from build123d import *

# Parameters (mm, degrees)
SKETCH1_W               = 6.35
SKETCH1_H               = 36.5125
CHAMFER2_SIZE           = 1.5875
SKETCH5_W               = 11.1125
SKETCH5_H               = 46.0375
CUT_EXTRUDE1_DEPTH      = 18.4625
CUT_EXTRUDE1_DEPTH_BACK = 18.4625
SKETCH6_R               = 12.3825
CUT_EXTRUDE2_DEPTH      = 7.3500001
CUT_EXTRUDE2_DEPTH_BACK = 7.3500001
SCALE1_SCALE            = 0.75
SCALE2_SCALE            = 0.666666667


with BuildPart() as part:
    # Sketch1 → Revolve1 (revolve)
    with BuildSketch(Plane.XY):
        with Locations((3.175, -18.25625)):
            Rectangle(SKETCH1_W, SKETCH1_H)
    revolve(axis=Axis((0, 46.0375, 0), (0, -1, 0)))

    # Chamfer2
    chamfer2_edges = [part.edges().sort_by_distance(p)[0] for p in [
        (-6.35, -36.5125, 0),
    ]]
    chamfer(chamfer2_edges, length=CHAMFER2_SIZE)

    # Sketch4 → Revolve2 (revolve)
    with BuildSketch(Plane.XY):
        with BuildLine():
            Line((6.35, 0), (0, 0))
            Line((0, 0), (0, 46.0375))
            ThreePointArc((0, 46.0375), (15.983688754, 35.607823052), (12.874497319, 16.77727882))
            ThreePointArc((12.874497319, 16.77727882), (8.03853042, 9.000640948), (6.35, 0))
        make_face()
    revolve(axis=Axis((0, 46.0375, 0), (0, 1, 0)))

    # Sketch5 → Cut-Extrude1 (cut, two sides)
    with BuildSketch(Plane(origin=(0, 0, 0), x_dir=(0, 0, -1), z_dir=(1, 0, 0))) as cut_extrude1_sk:
        with Locations((11.90625, 23.01875)):
            Rectangle(SKETCH5_W, SKETCH5_H)
        with Locations((-11.90625, 23.01875)):
            Rectangle(SKETCH5_W, SKETCH5_H)
    extrude(amount=CUT_EXTRUDE1_DEPTH, mode=Mode.SUBTRACT)
    extrude(cut_extrude1_sk.sketch, amount=-CUT_EXTRUDE1_DEPTH_BACK, mode=Mode.SUBTRACT)

    # Sketch6 → Cut-Extrude2 (cut, two sides)
    with BuildSketch(Plane.XY) as cut_extrude2_sk:
        with Locations((0, 28.575)):
            Circle(SKETCH6_R)
    extrude(amount=CUT_EXTRUDE2_DEPTH, mode=Mode.SUBTRACT)
    extrude(cut_extrude2_sk.sketch, amount=-CUT_EXTRUDE2_DEPTH_BACK, mode=Mode.SUBTRACT)


with BuildPart() as part_1:
    # Scale1: scaled about (-0.000122935, 7.334416679, -0.001044289)
    add(part.part.scale(SCALE1_SCALE).moved(Location((-3.0734e-05, 1.83360417, -0.000261072))))


with BuildPart() as part_2:
    # Scale2: scaled about (-0.000122935, 7.334416679, -0.001044289)
    add(part_1.part.scale(SCALE2_SCALE).moved(Location((-4.0978e-05, 2.44480556, -0.000348096))))


solid = part_2.part
Geometry: final body of the model. Coordinates: model frame, mm. A direction names the side the tool comes from. Give positions to 0.01 mm unless a question says otherwise; leave off trailing zeros. Loops run counter-clockwise (first coordinate to the right, second up) from the corner with the lowest first, then second, coordinate; pieces in that order, holes last. Notation, with made-up numbers: M 84,-26.5 L 90,-26.5 A27 ccw 90,5.5 Z; hole C -29,37 d2. An arc over 180 degrees is marked long. Put each result on its own line as item: value. Start each with the question number.
1) Ray query, line 1 along Y through (x, z) = (1.75, 0.5); line 2 along Y through (x, z) = (-5.25, -2.5); line 3 along X through (y, z) = (21.5, 3). Return the intervals inside material, ascending.
2) Cut plane B-B (y = 9). Output: boundary loops of the cut face in (x, z), then the cut area to 3 significant figures.
3) Contact query for a flat-ended pin moving along its axis: pin 1 (2 mm diameter, centred on x = 6, z = 1, fed in from +Y). Output: stop coordinate, or through.
4) Cut plane A-A (y = -6.5). Output: boundary loops of the cut face in (x, z) (3 decimals).
5) Access query for faces 1 (the flat face through (0, 11.5, -3.176)), 2 (the cylindrical face through (-0.69, -4.94, -3.1)). Directions: +Z, -Z, +X, -X, +Y, -Y. A direction counts if a zero-diameter tool reaches every point of the face in a straight line with its end or side. Return the directions, or none.
Verdict:
1. line 1: -14.59 to 12.02, 23.89 to 26.49
1. line 2: 11.32 to 14.67, 21.24 to 24.47
1. line 3: -7.39 to -5.08, 5.08 to 7.39
2. outline: M -3.02,-3.18 L 3.02,-3.18 A4.38 ccw 3.02,3.17 L -3.02,3.17 A4.38 ccw Z
2. area: 50.3 mm2
3. pin 1: y = 25.05
4. outline: C 0,-0.001 d6.35
5. face 1: -Z, +X, -X, +Y, -Y
5. face 2: -Y
